Verification items for the finished model (mm, model axes). A direction names the side the tool comes from. Coordinates: 2 decimals unless noted, no trailing zeros. Write each loop counter-clockwise with the first axis right and the second up, starting at its lowest first coordinate (ties: lowest second). Pieces come first, ordered by that corner, then holes. Notation, with made-up numbers: (83.25, -3) -> (106.25, -3) arc R12 ccw to (106.25, 11) -> close; hole circle Ø11 at (82.5, -23). An arc over 180 degrees is marked (long way). Answer in a Markdown table with one row per item.
```python
from build123d import *

# Parameters (mm, degrees)
SKETCH_1_W               = 20
SKETCH_1_H               = 18
EXTRUDE_1_DEPTH          = 25
SKETCH_2_W               = 16
SKETCH_2_H               = 14
CUT_EXTRUDE_1_DEPTH      = 21
CUT_EXTRUDE_2_DEPTH      = 32.320919527
CUT_EXTRUDE_2_DEPTH_BACK = 32.320919527
CUT_EXTRUDE_3_DEPTH      = 25.939927827
CUT_EXTRUDE_3_DEPTH_BACK = 25.939927827
CUT_EXTRUDE_4_DEPTH      = 32.016124839
CUT_EXTRUDE_4_DEPTH_BACK = 32.016124839
SKETCH_7_W               = 2
SKETCH_7_H               = 5
EXTRUDE_2_DEPTH          = 1
SKETCH_8_W               = 2
SKETCH_8_H               = 5
EXTRUDE_3_DEPTH          = 1


with BuildPart() as part:
    # 스케치1 → 보스-돌출1 (new body)
    with BuildSketch(Plane.XY):
        Rectangle(SKETCH_1_W, SKETCH_1_H)
    extrude(amount=EXTRUDE_1_DEPTH)

    # 스케치2 → 컷-돌출1 (cut)
    with BuildSketch(Plane.XY.offset(25)):
        with Locations((2, 0)):
            Rectangle(SKETCH_2_W, SKETCH_2_H)
    extrude(amount=-CUT_EXTRUDE_1_DEPTH, mode=Mode.SUBTRACT)

    # 스케치4 → 컷-돌출2 (cut, two sides: drawn at the far end of the back side and taken through both)
    with BuildSketch(Plane(origin=(0, -7, 0), x_dir=(1, 0, 0), z_dir=(0, 1, 0)).offset(-CUT_EXTRUDE_2_DEPTH_BACK)):
        Polygon((-6, -25), (10, -4), (10, -25), align=None)
    extrude(amount=CUT_EXTRUDE_2_DEPTH + CUT_EXTRUDE_2_DEPTH_BACK, mode=Mode.SUBTRACT)

    # 스케치5 → 컷-돌출3 (cut, two sides: drawn at the far end of the back side and taken through both)
    with BuildSketch(Plane.XY.offset(4).offset(-CUT_EXTRUDE_3_DEPTH_BACK)):
        with BuildLine():
            Line((-0.75, 2.75), (4.75, 2.75))
            ThreePointArc((4.75, 2.75), (7.5, 0), (4.75, -2.75))
            Line((4.75, -2.75), (-0.75, -2.75))
            ThreePointArc((-0.75, -2.75), (-3.5, 0), (-0.75, 2.75))
        make_face()
    extrude(amount=CUT_EXTRUDE_3_DEPTH + CUT_EXTRUDE_3_DEPTH_BACK, mode=Mode.SUBTRACT)

    # 스케치6 → 컷-돌출4 (cut, two sides: drawn at the far end of the back side and taken through both)
    with BuildSketch(Plane(origin=(-6, 0, 0), x_dir=(0, 0, -1), z_dir=(1, 0, 0)).offset(-CUT_EXTRUDE_4_DEPTH_BACK)):
        with BuildLine():
            Line((-17.25, 2.75), (-11.75, 2.75))
            ThreePointArc((-11.75, 2.75), (-9, 0), (-11.75, -2.75))
            Line((-11.75, -2.75), (-17.25, -2.75))
            ThreePointArc((-17.25, -2.75), (-20, 0), (-17.25, 2.75))
        make_face()
    extrude(amount=CUT_EXTRUDE_4_DEPTH + CUT_EXTRUDE_4_DEPTH_BACK, mode=Mode.SUBTRACT)

    # 스케치7 → 보스-돌출2 (add)
    with BuildSketch(Plane(origin=(0, 0, 0), x_dir=(-1, 0, 0), z_dir=(0, 0, -1))):
        with Locations((-8.8, 0)):
            Rectangle(SKETCH_7_W, SKETCH_7_H)
        with Locations((8.8, 0)):
            Rectangle(SKETCH_7_W, SKETCH_7_H)
    extrude(amount=EXTRUDE_2_DEPTH)

    # 스케치8 → 보스-돌출3 (add)
    with BuildSketch(Plane.ZY.offset(10)):
        with Locations((1.2, 0)):
            Rectangle(SKETCH_8_W, SKETCH_8_H)
        with Locations((23.8, 0)):
            Rectangle(SKETCH_8_W, SKETCH_8_H)
    extrude(amount=EXTRUDE_3_DEPTH)


solid = part.part
```
1. Section check D-D, the plane y = 3.5. Record the boundary of the cut face in (x, z).
Geometry says:
| item | result |
|---|---|
| outline | (-10, 0) -> (10, 0) -> (10, 4) -> (-6, 4) -> (-6, 25) -> (-10, 25) -> close |
2. Depth check by flat-ended pin: P1, Ø1.1, axis at y = -0.5, z = -0.5, coming from the +X side; P2, Ø8, axis at x = -8.5, y = -7, coming from the -Z side; P3, Ø1.1, axis at y = -0.5, z = -0.5, coming from the -X side; P4, Ø7, axis at x = 2.5, y = 2.5, coming from the +Z side. Enter the tip coordinate at first touch or a pass-through.
Geometry says:
| item | result |
|---|---|
| P1 | x = 10 |
| P2 | z = 0 |
| P3 | x = -10 |
| P4 | z = 4 |
3. Section check B-B, the plane x = 5.5. Record the boundary of the cut face in (y, z), plus the area to 3 significant figures.
Geometry says:
| item | result |
|---|---|
| outline | (-9, 0) -> (-2.65, 0) -> (-2.65, 4) -> (-7, 4) -> (-7, 9.91) -> (-9, 9.91) -> close; (2.65, 0) -> (9, 0) -> (9, 9.91) -> (7, 9.91) -> (7, 4) -> (2.65, 4) -> close |
| area | 74.5 mm^2 |
4. Tool access check on faces 1 (the flat face through (-10.5, -2.5, 23.8)), 2 (the cylindrical face through (7.5, 0.1, 2)), 3 (the flat face through (-6, 3, 15)). Record the directions out of +Z, -Z, +X, -X, +Y, -Y that give a thin tool (end or side, any length) a straight path to the whole face; none if there is none.
Geometry says:
| item | result |
|---|---|
| face 1 | +Z, -Z, -X, -Y |
| face 2 | +Z, -Z |
| face 3 | +Z, +X |
5. Section check C-C, the plane z = 16. Record the boundary of the cut face in (x, y).
Geometry says:
| item | result |
|---|---|
| outline | (-10, -9) -> (0.86, -9) -> (0.86, -7) -> (-6, -7) -> (-6, -2.75) -> (-10, -2.75) -> close; (-10, 2.75) -> (-6, 2.75) -> (-6, 7) -> (0.86, 7) -> (0.86, 9) -> (-10, 9) -> close |
6. Thickness scan on line 1 (Y direction, x = -3, z = 11.5); line 2 (X direction, y = -3.75, z = 20.75); line 3 (Z direction, x = -4.5, y = 1.75). Record the ranges inside material, lowest first. Write a range as from..to.
Geometry says:
| item | result |
|---|---|
| line 1 | -9..-7, 7..9 |
| line 2 | -10..-6 |
| line 3 | 0..4 |
7. Section check A-A, the plane y = 0. State how many separate pieces and enclosed holes the cut face has, plus the area to 3 significant figures.
Geometry says:
| item | result |
|---|---|
| separate pieces | 3 |
| enclosed holes | 0 |
| area | 84.0 mm^2 |
8. Mould release check, pull along Z, two halves, no side actions. Record for faces 4 (the flat face through (2, -3, 4)), 5 (the cylindrical face through (-8, 0, 9)), 6 (the flat face through (7.8, 0, -0.5)): released by +Z, released by -Z, zero draft, split by the parting line, or undercut.
Geometry says:
| item | result |
|---|---|
| face 4 | released by +Z |
| face 5 | undercut |
| face 6 | zero draft |
